CAD build for the part. Positions are in the model's coordinates, mm. Face numbers are marked on the shaded views. A direction names the side the tool comes from. Give positions to 0.01 mm unless a question says otherwise; leave off trailing zeros. Loops run counter-clockwise (first coordinate to the right, second up) from the corner with the lowest first, then second, coordinate; pieces in that order, holes last. Notation, with made-up numbers: M 76.25,24.5 L 134.25,24.5 A21 cw 134.25,39.5 Z; hole C 80,57 d11. An arc over 180 degrees is marked long. Answer as CSV lines item,"result".
```python
from build123d import *

# Parameters (mm, degrees)
SKETCH2_W                      = 40
SKETCH2_H                      = 31.916671008
BOSS_EXTRUDE1_DEPTH            = 20
CBORE_FOR_M5_SHCS1_D           = 5.5
CBORE_FOR_M5_SHCS1_CBORE_D     = 10
CBORE_FOR_M5_SHCS1_CBORE_DEPTH = 25
M5X0_8_TAPPED_HOLE1_D          = 4.2
FILLET1_R                      = 22
FILLET2_START                  = -21
FILLET2_DEPTH                  = 22


with BuildPart() as part:
    # Sketch2 → Boss-Extrude1 (new body)
    with BuildSketch(Plane(origin=(0, 0, 0), x_dir=(1, 0, 0), z_dir=(0, 1, 0))):
        with Locations((2.27, -10.958335504)):
            Rectangle(SKETCH2_W, SKETCH2_H)
    extrude(amount=-BOSS_EXTRUDE1_DEPTH)

    # CBORE for M5 SHCS1 (through all)
    with Locations(Plane.XY.offset(26.916671008)):
        with Locations((-10.23, -10), (12.27, -10)):
            CounterBoreHole(CBORE_FOR_M5_SHCS1_D / 2, CBORE_FOR_M5_SHCS1_CBORE_D / 2, CBORE_FOR_M5_SHCS1_CBORE_DEPTH)

    # M5x0.8 Tapped Hole1 (through all)
    with Locations(Plane(origin=(0, 0, 0), x_dir=(1, 0, 0), z_dir=(0, 1, 0))):
        with Locations((-1.73, -17.916671008), (0, 0)):
            Hole(M5X0_8_TAPPED_HOLE1_D / 2)

    # Fillet1
    # the kernel refuses this fillet: 22 mm, written as the material it takes off along each edge
    with BuildSketch(Plane(origin=(22.27, 55, 26.916671008), x_dir=(0, 0, -1), z_dir=(0, -1, 0))) as fillet1_piece_1:
        with BuildLine():
            CenterArc((FILLET1_R, -FILLET1_R), FILLET1_R, 90, 90)
            Line((0, -FILLET1_R), (0, 0))
            Line((0, 0), (FILLET1_R, 0))
        make_face()
    extrude(amount=130, mode=Mode.SUBTRACT)

    # Fillet2: read off the stored shape, not the designer's step
    # Fillet2 outline → Fillet2 (cut)
    with BuildSketch(Plane(origin=(0, 0, 0), x_dir=(1, 0, 0), z_dir=(0, 1, 0)).offset(FILLET2_START)):
        with BuildLine():
            ThreePointArc((-7.73, -26.916671008), (-14.801067812, -23.98773882), (-17.73, -16.916671008))
            Line((-17.73, -16.916671008), (-17.73, -26.916671008))
            Line((-17.73, -26.916671008), (-7.73, -26.916671008))
        make_face()
    extrude(amount=FILLET2_DEPTH, mode=Mode.SUBTRACT)


solid = part.part
```
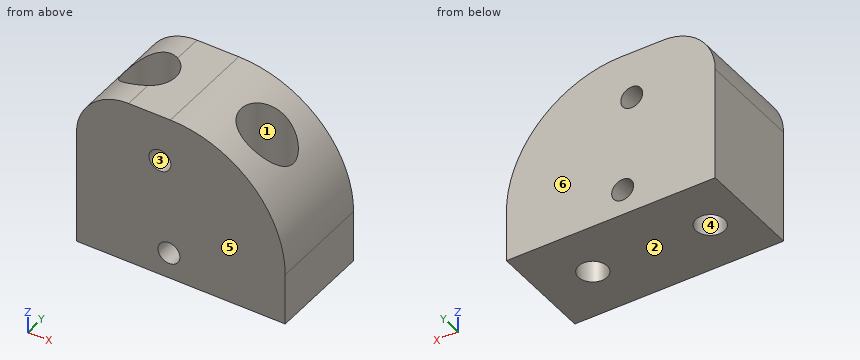
Q1. Cut at D-D (z = 22). Write the cut outline in (x, y), and give its area (3 significant figures).
Solution:
outline,"M -16.34,-20 L 14.13,-20 L 14.13,-14.64 A5 cw long 14.13,-5.36 L 14.13,0 L -16.34,0 Z; hole C -10.23,-10 d10"
area,"473 mm²"
Q2. Which spindle directions (+Z, -Z, +X, -X, +Y, -Y) get a long thin tool onto all of the face, cutting with end or side? Do the marked faces 1 and 2. Say none if no direction does.
Solution:
face 1,"+Z"
face 2,"-Z, +X, -X, +Y, -Y"
Q3. Cut at A-A (z = 0). Write the cut outline in (x, y), and give its area (3 significant figures).
Solution:
outline,"M -17.73,-20 L -2.1,-20 L -2.1,0 L -17.73,0 Z; M 2.1,-20 L 22.27,-20 L 22.27,0 L 2.1,0 Z; hole C -10.23,-10 d5.5; hole C 12.27,-10 d5.5"
area,"668 mm²"
Q4. Pin check, flat tips, straight feed: P1, Ø4.5, axis at x = -10.23, y = -10, coming from the -Z side; P2, Ø3, axis at y = -14, z = 13, coming from the +X side; P3, Ø8, axis at x = 12.5, y = -12.5, coming from the +Z side; P4, Ø5, axis at x = -10.5, y = -10.5, coming from the +Z side. Stop position of each tip, or through.
Solution:
P1,"passes through"
P2,"stops at x = 21.26"
P3,"stops at z = 25.28"
P4,"stops at z = 1.92"
Q5. Wall check: line 1 (Y direction, x = 12.27, z = 14.75); line 2 (Z direction, x = -0.5, y = -15.5); line 3 (X direction, y = -7.75, z = 8.5). Give the ranges that are in metal, low to high. Write a range as [from, to].
Solution:
line 1,"y = [-20, -15], [-5, 0]"
line 2,"z = [-5, -2.04], [2.04, 16.21], [19.62, 26.92]"
line 3,"x = [-17.73, -14.7], [-5.76, 7.8], [16.74, 21.98]"
Q6. Cut at B-B (y = -12). Write the cut outline in (x, z).
Solution:
outline,"M -17.73,-5 L -12.12,-5 L -12.12,1.92 L -14.81,1.92 L -14.81,23.98 A10 ccw -17.73,16.92 Z; M -8.34,-5 L 10.38,-5 L 10.38,1.92 L 7.69,1.92 L 7.69,25.63 A22 ccw 0.27,26.92 L -5.65,26.92 L -5.65,1.92 L -8.34,1.92 Z; M 14.16,-5 L 22.27,-5 L 22.27,4.92 A22 ccw 16.85,19.37 L 16.85,1.92 L 14.16,1.92 Z; hole C -1.73,17.92 d4.2; hole C 0,0 d4.2"
Q7. Mould opens along Y. For the marked faces 3, 4, 5 and 6 say: released by +Y, released by -Y, zero draft, split by the parting line, or undercut.
Solution:
face 3,"zero draft"
face 4,"undercut"
face 5,"released by -Y"
face 6,"released by +Y"
Q8. Cut at C-C (x = 12.27). Write the cut outline in (y, z).
Solution:
outline,"M -20,-5 L -12.75,-5 L -12.75,1.92 L -15,1.92 L -15,23.36 L -20,23.36 Z; M -7.25,-5 L 0,-5 L 0,23.36 L -5,23.36 L -5,1.92 L -7.25,1.92 Z"
